```python
from build123d import *

# Parameters (mm, degrees)
BOSS_EXTRUDE1_DEPTH      = 25
BOSS_EXTRUDE1_DEPTH_BACK = 25
CUT_EXTRUDE2_DEPTH       = 87.168439698
CUT_EXTRUDE2_DEPTH_BACK  = 87.168439698
SKETCH3_W                = 27.604398764
SKETCH3_H                = 36.5
CUT_EXTRUDE3_DEPTH       = 87.168439698
CUT_EXTRUDE3_DEPTH_BACK  = 87.168439698
SKETCH4_R                = 1.47496879


with BuildPart() as part:
    # Sketch1 → Boss-Extrude1 (new, two sides: drawn at the far end of the back side and taken through both)
    with BuildSketch(Plane(origin=(0, 0, 0), x_dir=(1, 0, 0), z_dir=(0, 1, 0)).offset(-BOSS_EXTRUDE1_DEPTH_BACK)):
        with BuildLine():
            Line((0, -20), (-80, -20))
            Line((-80, -20), (-80, 20))
            Line((-80, 20), (0, 20))
            ThreePointArc((0, 20), (5.358983849, 0), (0, -20))
        make_face()
    extrude(amount=BOSS_EXTRUDE1_DEPTH + BOSS_EXTRUDE1_DEPTH_BACK)

    # Sketch3 → Cut-Extrude2 (cut, two sides: drawn at the far end of the back side and taken through both)
    with BuildSketch(Plane.XY.offset(-CUT_EXTRUDE2_DEPTH_BACK)):
        with Locations((-5.838816769, 0)):
            Rectangle(SKETCH3_W, SKETCH3_H)
    extrude(amount=CUT_EXTRUDE2_DEPTH + CUT_EXTRUDE2_DEPTH_BACK, mode=Mode.SUBTRACT)

    # Sketch4 → Cut-Extrude3 (cut, two sides: drawn at the far end of the back side and taken through both)
    with BuildSketch(Plane(origin=(0, 0, 0), x_dir=(1, 0, 0), z_dir=(0, 1, 0)).offset(-CUT_EXTRUDE3_DEPTH_BACK)):
        with Locations(Location((-7.141016151, 0, 0), (0, 0, 270))):
            Circle(SKETCH4_R)
    extrude(amount=CUT_EXTRUDE3_DEPTH + CUT_EXTRUDE3_DEPTH_BACK, mode=Mode.SUBTRACT)


solid = part.part
```
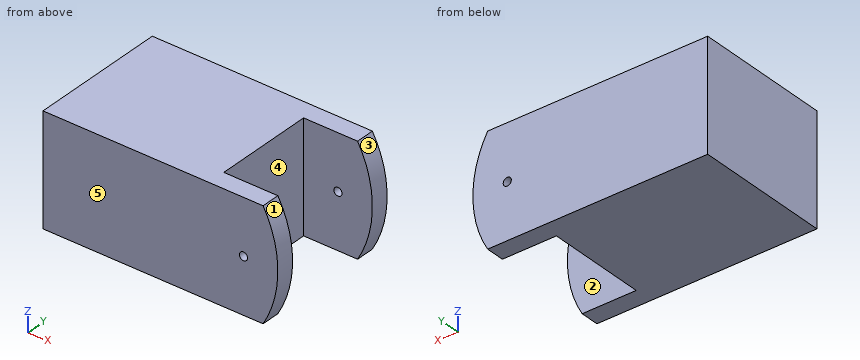
Can you work these out from the model? Positions are in its coordinate system, mm. Face numbers are marked on the shaded views. A direction names the side the tool comes from. Give positions to 0.01 mm unless a question says otherwise; leave off trailing zeros. Loops run counter-clockwise (first coordinate to the right, second up) from the corner with the lowest first, then second, coordinate; pieces in that order, holes last. Notation, with made-up numbers: M 45,19.25 L 77,19.25 A12 cw 77,41.25 Z; hole C -30.75,-10.75 d9. An arc over 180 degrees is marked long. Answer in a Markdown table with one row per item.
1. Thinking about a two-plate mould opening in Y: for the marked faces 3, 4 and 5, which applies, released by +Y, released by -Y, zero draft, split by the parting line, or undercut?
Taken from the geometry:
| item | result |
|---|---|
| face 3 | zero draft |
| face 4 | undercut |
| face 5 | released by -Y |
2. Suppose I cut it at A-A on z = 0. Write out the boundary of the cut face in (x, y).
Taken from the geometry:
| item | result |
|---|---|
| outline | M -80,-25 L -8.62,-25 L -8.62,-18.25 L -19.64,-18.25 L -19.64,18.25 L -8.62,18.25 L -8.62,25 L -80,25 Z; M -5.67,-25 L 5.36,-25 L 5.36,-18.25 L -5.67,-18.25 Z; M -5.67,18.25 L 5.36,18.25 L 5.36,25 L -5.67,25 Z |
3. If I drill on line 1 along Y through (x, z) = (-19.5, -6); line 2 along X through (y, z) = (-23.5, 0); line 3 along X through (y, z) = (-5.5, 16), over which ranges is the centre line in solid material (lowest first)?
Taken from the geometry:
| item | result |
|---|---|
| line 1 | y = -25 to -18.25, 18.25 to 25 |
| line 2 | x = -80 to -8.62, -5.67 to 5.36 |
| line 3 | x = -80 to -19.64 |
4. Which directions (+Z, -Z, +X, -X, +Y, -Y) give clear straight access to the entire face, cutting with the end or side of a thin tool? Please do the marked faces 1 and 2.
Taken from the geometry:
| item | result |
|---|---|
| face 1 | +X, +Y, -Y |
| face 2 | +Z, -Z, +X |
5. Suppose I cut it at B-B on y = 22. Write out the boundary of the cut face in (x, z), plus the area to 3 significant figures.
Taken from the geometry:
| item | result |
|---|---|
| outline | M -80,-20 L 0,-20 A40 ccw 0,20 L -80,20 Z; hole C -7.14,0 d2.95 |
| area | 3,340 mm² |
6. For pin 1 Ø2.5 at (x, z) = (-7.14, 0) entering from +Y; pin 2 Ø4 at (x, z) = (-7.14, 0) entering from -Y; pin 3 Ø1.5 at (y, z) = (7.5, -15.5) entering from +X, each with a flat end and sliding along its axis, tell me the tip position at first contact or that it passes through.
Taken from the geometry:
| item | result |
|---|---|
| pin 1 | passes through |
| pin 2 | stops at y = -25 |
| pin 3 | stops at x = -19.64 |
7. Suppose I cut it at C-C on z = -17. Write out the boundary of the cut face in (x, y).
Taken from the geometry:
| item | result |
|---|---|
| outline | M -80,-25 L 1.57,-25 L 1.57,-18.25 L -19.64,-18.25 L -19.64,18.25 L 1.57,18.25 L 1.57,25 L -80,25 Z |
8. Suppose I cut it at D-D on y = -2.5. Write out the boundary of the cut face in (x, z), plus the area to 3 significant figures.
Taken from the geometry:
| item | result |
|---|---|
| outline | M -80,-20 L -19.64,-20 L -19.64,20 L -80,20 Z |
| area | 2,410 mm² |
